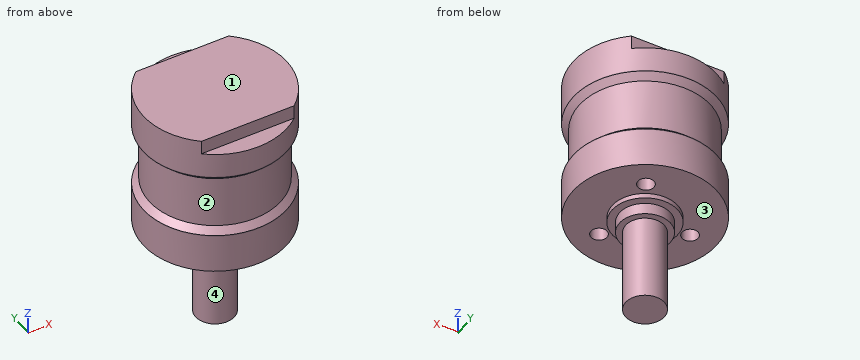
from build123d import *

# Parameters (mm, degrees)
SKETCH1_R           = 11.1125
BOSS_EXTRUDE1_DEPTH = 6.096
SKETCH2_R           = 10.16
BOSS_EXTRUDE2_DEPTH = 10.16
SKETCH3_R           = 11.1125
BOSS_EXTRUDE3_DEPTH = 6.096
CUT_EXTRUDE1_START  = -2.159
CUT_EXTRUDE1_DEPTH  = 2.159
CHAMFER1_SIZE       = 1.016
SKETCH5_R           = 5.08
BOSS_EXTRUDE4_DEPTH = 0.762
SKETCH6_R           = 3.937
BOSS_EXTRUDE5_DEPTH = 1.778
SKETCH7_R           = 2.9972
BOSS_EXTRUDE6_DEPTH = 13.335
SKETCH8_R           = 1.25
CUT_EXTRUDE2_DEPTH  = 7.747


with BuildPart() as part:
    # Sketch1 → Boss-Extrude1 (new body)
    with BuildSketch(Plane.XY):
        with Locations(Location((0, 0, 0), (0, 0, 180))):
            Circle(SKETCH1_R)
    extrude(amount=BOSS_EXTRUDE1_DEPTH)

    # Sketch2 → Boss-Extrude2 (add)
    with BuildSketch(Plane.XY.offset(6.096)):
        Circle(SKETCH2_R)
    extrude(amount=BOSS_EXTRUDE2_DEPTH)

    # Sketch3 → Boss-Extrude3 (add)
    with BuildSketch(Plane.XY.offset(16.256)):
        with Locations(Location((0, 0, 0), (0, 0, 180))):
            Circle(SKETCH3_R)
    extrude(amount=BOSS_EXTRUDE3_DEPTH)

    # Sketch4 → Cut-Extrude1 (cut)
    with BuildSketch(Plane.XY.offset(22.352).offset(CUT_EXTRUDE1_START)):
        with BuildLine():
            ThreePointArc((7.207392664, 8.4582), (0, 11.1125), (-7.207392664, 8.4582))
            Line((-7.207392664, 8.4582), (7.207392664, 8.4582))
        make_face()
        with BuildLine():
            Line((7.207392664, -8.4582), (-7.207392664, -8.4582))
            ThreePointArc((-7.207392664, -8.4582), (0, -11.1125), (7.207392664, -8.4582))
        make_face()
    extrude(amount=CUT_EXTRUDE1_DEPTH, mode=Mode.SUBTRACT)

    # Chamfer1
    # the kernel refuses this chamfer: 1.016 mm, written as the material it adds along each edge
    with BuildSketch(Plane(origin=(0, 0, 6.096), x_dir=(1, 0, 0), z_dir=(0, -1, 0))) as chamfer1_piece_1_section:
        Polygon((10.16, CHAMFER1_SIZE), (10.16 + CHAMFER1_SIZE, 0), (10.16, 0), align=None)
    chamfer1_piece_1 = revolve(axis=Axis((0, 0, 6.096), (0, 0, 1)), mode=Mode.PRIVATE)
    chamfer1_piece_1 = chamfer1_piece_1 & Plane(origin=(0, 0, 6.626545895), x_dir=(-1, 0, 0), z_dir=(0, 0, -1)) * Cylinder(11.1125, 45, mode=Mode.PRIVATE)
    add(chamfer1_piece_1)
    with BuildSketch(Plane(origin=(0, 0, 16.256), x_dir=(1, 0, 0), z_dir=(0, -1, 0))) as chamfer1_piece_2_section:
        Polygon((10.16 + CHAMFER1_SIZE, 0), (10.16, -CHAMFER1_SIZE), (10.16, 0), align=None)
    chamfer1_piece_2 = revolve(axis=Axis((0, 0, 16.256), (0, 0, 1)), mode=Mode.PRIVATE)
    chamfer1_piece_2 = chamfer1_piece_2 & Plane(origin=(0, 0, 15.725454105), x_dir=(-1, 0, 0), z_dir=(0, 0, -1)) * Cylinder(11.1125, 45, mode=Mode.PRIVATE)
    add(chamfer1_piece_2)

    # Sketch5 → Boss-Extrude4 (add)
    with BuildSketch(Plane(origin=(0, 0, 0), x_dir=(-1, 0, 0), z_dir=(0, 0, -1))):
        with Locations(Location((0, 0, 0), (0, 0, 180))):
            Circle(SKETCH5_R)
    extrude(amount=BOSS_EXTRUDE4_DEPTH)

    # Sketch6 → Boss-Extrude5 (add)
    with BuildSketch(Plane(origin=(0, 0, -0.762), x_dir=(-1, 0, 0), z_dir=(0, 0, -1))):
        Circle(SKETCH6_R)
    extrude(amount=BOSS_EXTRUDE5_DEPTH)

    # Sketch7 → Boss-Extrude6 (add)
    with BuildSketch(Plane(origin=(0, 0, -2.54), x_dir=(-1, 0, 0), z_dir=(0, 0, -1))):
        Circle(SKETCH7_R)
    extrude(amount=BOSS_EXTRUDE6_DEPTH)

    # Sketch8 → Cut-Extrude2 (cut)
    with BuildSketch(Plane(origin=(0, 0, 0), x_dir=(-1, 0, 0), z_dir=(0, 0, -1))):
        with Locations((7, 0)):
            Circle(SKETCH8_R)
        with Locations((-3.5, -6.062177826)):
            Circle(SKETCH8_R)
        with Locations((-3.5, 6.062177826)):
            Circle(SKETCH8_R)
    extrude(amount=-CUT_EXTRUDE2_DEPTH, mode=Mode.SUBTRACT)


solid = part.part
Design review of the part built by this model. Coordinates are the model's own, in mm. Face numbers are marked on the shaded views. Coordinates: 2 decimals unless noted, no trailing zeros. Order: outer loops, then holes, each group sorted by start corner. A loop starts at its lowest first (then second) coordinate and runs counter-clockwise, first axis right, second up.
Item 1: The part is to be moulded in two halves that separate along Z. For the marked faces 1, 2, 3 and 4, say which applies: pulls with the +Z half, pulls with the -Z half, needs draft (parallel to the pull), parting line crosses it, or undercut.
Item 2: Take a section at D-D, the plane z = 19.5. Write out the cut boundary in (x, y) (1 decimal), then the cut area to 3 significant figures.
Item 3: For line 1 (Y direction, x = 3.5, z = 2.5); line 2 (Z direction, x = 8.25, y = 0.75); line 3 (X direction, y = -0.5, z = 2), list the stretches that pass through material, from the lowest coordinate up.
Item 4: For pin 1 Ø1.1 at (x, z) = (-3.5, 21) entering from +Y; pin 2 Ø8 at (y, z) = (8, 5) entering from +X; pin 3 Ø3 at (x, y) = (-7, 0) entering from -Z; pin 4 Ø2 at (x, z) = (-5.5, -4.5) entering from -Y, all flat-tipped, find the tip position at first contact; note any pin that passes through.
Item 5: Take a section at C-C, the plane z = 12.5. Write out the cut boundary in (x, y).
Item 6: Take a section at B-B, the plane x = 0. Write out the cut boundary in (y, z) (1 decimal), then the cut area to 3 significant figures.
The answers:
1. face 1: pulls with the +Z half
1. face 2: undercut
1. face 3: pulls with the -Z half
1. face 4: needs draft
2. outline: circle Ø22.2 at (0, 0)
2. area: 388 mm2
3. line 1: y = -10.55 to -7.31, -4.81 to 4.81, 7.31 to 10.55
3. line 2: z = 0 to 22.35
3. line 3: x = -11.1 to -8.15, -5.85 to 11.1
4. pin 1: stops at y = 8.46
4. pin 2: stops at x = 10.37
4. pin 3: stops at z = 0
4. pin 4: passes through
5. outline: circle Ø20.32 at (0, 0)
6. outline: (-11.1, 0) - (-5.1, 0) - (-5.1, -0.8) - (-3.9, -0.8) - (-3.9, -2.5) - (-3, -2.5) - (-3, -15.9) - (3, -15.9) - (3, -2.5) - (3.9, -2.5) - (3.9, -0.8) - (5.1, -0.8) - (5.1, 0) - (11.1, 0) - (11.1, 6.2) - (10.2, 7.1) - (10.2, 15.2) - (11.1, 16.2) - (11.1, 20.2) - (8.5, 20.2) - (8.5, 22.4) - (-8.5, 22.4) - (-8.5, 20.2) - (-11.1, 20.2) - (-11.1, 16.2) - (-10.2, 15.2) - (-10.2, 7.1) - (-11.1, 6.2) - close
6. area: 570 mm2
